```python
from build123d import *

# Parameters (mm, degrees)
SKETCH1_W           = 65
SKETCH1_H           = 65
BOSS_EXTRUDE1_DEPTH = 4
SKETCH2_R           = 1.55
SKETCH2_R_2         = 11.25
CUT_EXTRUDE1_DEPTH  = 4
SKETCH3_W           = 10
SKETCH3_H           = 4
SKETCH3_W_2         = 15
CUT_EXTRUDE2_DEPTH  = 4
SKETCH5_W           = 4
SKETCH5_H           = 6
SKETCH5_H_2         = 15
CUT_EXTRUDE3_DEPTH  = 4
SKETCH6_R           = 1.55
SKETCH6_R_2         = 4
CUT_EXTRUDE4_DEPTH  = 4


with BuildPart() as part:
    # Sketch1 → Boss-Extrude1 (new body)
    with BuildSketch(Plane(origin=(0, 0, 0), x_dir=(0, 0, -1), z_dir=(1, 0, 0))):
        with Locations((32.5, 32.5)):
            Rectangle(SKETCH1_W, SKETCH1_H)
    extrude(amount=BOSS_EXTRUDE1_DEPTH)

    # Sketch2 → Cut-Extrude1 (cut)
    with BuildSketch(Plane(origin=(4, 0, 0), x_dir=(0, 0, -1), z_dir=(1, 0, 0))):
        with Locations((17, 48)):
            Circle(SKETCH2_R)
        with Locations((32.5, 32.5)):
            Circle(SKETCH2_R_2)
        with Locations((48, 48)):
            Circle(SKETCH2_R)
        with Locations((48, 17)):
            Circle(SKETCH2_R)
        with Locations((17, 17)):
            Circle(SKETCH2_R)
    extrude(amount=-CUT_EXTRUDE1_DEPTH, mode=Mode.SUBTRACT)

    # Sketch3 → Cut-Extrude2 (cut)
    with BuildSketch(Plane(origin=(4, 0, 0), x_dir=(0, 0, -1), z_dir=(1, 0, 0))):
        with Locations((5, 63)):
            Rectangle(SKETCH3_W, SKETCH3_H)
        with Locations((32.5, 63)):
            Rectangle(SKETCH3_W_2, SKETCH3_H)
        with Locations((60, 63)):
            Rectangle(SKETCH3_W, SKETCH3_H)
        with Locations((60, 2)):
            Rectangle(SKETCH3_W, SKETCH3_H)
        with Locations((32.5, 2)):
            Rectangle(SKETCH3_W_2, SKETCH3_H)
        with Locations((5, 2)):
            Rectangle(SKETCH3_W, SKETCH3_H)
    extrude(amount=-CUT_EXTRUDE2_DEPTH, mode=Mode.SUBTRACT)

    # Sketch5 → Cut-Extrude3 (cut)
    with BuildSketch(Plane(origin=(4, 0, 0), x_dir=(0, 0, -1), z_dir=(1, 0, 0))):
        with Locations((2, 58)):
            Rectangle(SKETCH5_W, SKETCH5_H)
        with Locations((2, 32.5)):
            Rectangle(SKETCH5_W, SKETCH5_H_2)
        with Locations((2, 7)):
            Rectangle(SKETCH5_W, SKETCH5_H)
        with Locations((63, 7)):
            Rectangle(SKETCH5_W, SKETCH5_H)
        with Locations((63, 32.5)):
            Rectangle(SKETCH5_W, SKETCH5_H_2)
        with Locations((63, 58)):
            Rectangle(SKETCH5_W, SKETCH5_H)
    extrude(amount=-CUT_EXTRUDE3_DEPTH, mode=Mode.SUBTRACT)

    # Sketch6 → Cut-Extrude4 (cut)
    with BuildSketch(Plane(origin=(4, 0, 0), x_dir=(0, 0, -1), z_dir=(1, 0, 0))):
        with Locations((7.5, 37.5)):
            Circle(SKETCH6_R)
        with Locations((17.5, 37.5)):
            Circle(SKETCH6_R)
        with Locations((17.5, 27.5)):
            Circle(SKETCH6_R)
        with Locations((12.5, 32.5)):
            Circle(SKETCH6_R_2)
        with Locations((7.5, 27.5)):
            Circle(SKETCH6_R)
        with Locations((52.5, 32.5)):
            Circle(SKETCH6_R_2)
        with Locations((47.5, 27.5)):
            Circle(SKETCH6_R)
        with Locations((47.5, 37.5)):
            Circle(SKETCH6_R)
        with Locations((57.5, 37.5)):
            Circle(SKETCH6_R)
        with Locations((57.5, 27.5)):
            Circle(SKETCH6_R)
    extrude(amount=-CUT_EXTRUDE4_DEPTH, mode=Mode.SUBTRACT)


solid = part.part
```
Input: part model. Units: mm. Frame: model coordinates. A direction names the side the tool comes from. Give positions to 0.01 mm unless a question says otherwise; leave off trailing zeros. Order: outer loops, then holes, each group sorted by start corner. A loop starts at its lowest first (then second) coordinate and runs counter-clockwise, first axis right, second up. Notation, with made-up numbers: (66, 77) - (99, 77) arc R23 cw to (99, 109) - close; hole circle Ø10 at (50.25, 66). An arc over 180 degrees is marked (long way). One line per item, written item: value.
1. Cut plane C-C, the plane y = 27.5. Output: boundary loops of the cut face in (x, z), and give its area (3 significant figures).
Determined:
outline: (0, -61) - (4, -61) - (4, -59.05) - (0, -59.05) - close; (0, -55.95) - (4, -55.95) - (4, -49.05) - (0, -49.05) - close; (0, -45.95) - (4, -45.95) - (4, -42.58) - (0, -42.58) - close; (0, -22.42) - (4, -22.42) - (4, -19.05) - (0, -19.05) - close; (0, -15.95) - (4, -15.95) - (4, -9.05) - (0, -9.05) - close; (0, -5.95) - (4, -5.95) - (4, -4) - (0, -4) - close
area: 97.8 mm2
2. Cut plane A-A, the plane y = 17. Output: boundary loops of the cut face in (x, z), and give its area (3 significant figures).
Determined:
outline: (0, -65) - (4, -65) - (4, -49.55) - (0, -49.55) - close; (0, -46.45) - (4, -46.45) - (4, -18.55) - (0, -18.55) - close; (0, -15.45) - (4, -15.45) - (4, 0) - (0, 0) - close
area: 235 mm2
3. Cut plane B-B, the plane z = -32.5. Output: boundary loops of the cut face in (x, y), and give its area (3 significant figures).
Determined:
outline: (0, 4) - (4, 4) - (4, 21.25) - (0, 21.25) - close; (0, 43.75) - (4, 43.75) - (4, 61) - (0, 61) - close
area: 138 mm2
4. Cut plane D-D, the plane x = 2.1. Give the number of separate pieces and of enclosed holes in the cut face, and give its area (3 significant figures).
Determined:
separate pieces: 1
enclosed holes: 15
area: 3,140 mm2
5. Reachability of faces 4 (the face through (2, 2, -25)), 5 (the face through (2, 7, -61)), 6 (the face through (2, 58, -61)), 7 (the face through (2, 7, -4)), 8 (the face through (2, 61, -7)) from +Z, -Z, +X, -X, +Y, -Y: full face, straight path, thin tool, end or side. Return the list, or none.
Determined:
face 4: +X, -X, -Y
face 5: -Z, +X, -X, -Y
face 6: -Z, +X, -X, +Y
face 7: +Z, +X, -X, -Y
face 8: +Z, +X, -X, +Y
6. Line query: probe 1 along Y at (x, z) = (1.8, -57.5); probe 2 along Z at (x, y) = (0.2, 62); probe 3 along Z at (x, y) = (1.35, 28). Output: solid intervals per line, ascending.
Determined:
probe 1: 4 to 25.95, 29.05 to 35.95, 39.05 to 61
probe 2: -55 to -40, -25 to -10
probe 3: -61 to -58.97, -56.03 to -48.97, -46.03 to -42.81, -22.19 to -18.97, -16.03 to -8.97, -6.03 to -4
7. Draft query along Y for faces 1 (the face through (2, 65, -47)), 2 (the face through (2, 58, -4)), 3 (the face through (2, 40, -2)). Return one class per face: released by +Y, released by -Y, zero draft, split by the parting line, or undercut.
Determined:
face 1: released by +Y
face 2: zero draft
face 3: undercut
8. Pin query (flat end, axial travel): pin 1 Ø2 at (x, y) = (1.5, 57.5) entering from +Z; pin 2 Ø2 at (x, z) = (3, -62.5) entering from +Y. Return the tip coordinate at first contact, or that it passes through.
Determined:
pin 1: z = -4
pin 2: y = 55
